Source: CAD feature listing. Evaluate the final solid. Frame: model axes, mm. A direction names the side the tool comes from. Coordinates: 2 decimals unless noted, no trailing zeros. Order: outer loops, then holes, each group sorted by start corner. A loop starts at its lowest first (then second) coordinate and runs counter-clockwise, first axis right, second up.
```python
from build123d import *

# Parameters (mm, degrees)
F0_W      = 72
F0_H      = 24.5
F1_DEPTH  = 18.5
F3_DEPTH  = 11
F3_FACE_R = 14.75
F4_DEPTH  = 19.5
F5_W      = 72
F5_H      = 24.5
F6_DEPTH  = 22.945
F8_DEPTH  = 52.5


with BuildPart() as f1:
    # F0 (on Top) → F1 (new body)
    with BuildSketch(Plane.XY):
        with Locations((36, 12.25)):
            Rectangle(F0_W, F0_H)
    extrude(amount=F1_DEPTH)

    # F2 (on face) → F3 (join)
    with BuildSketch(Plane.YZ.offset(72)):
        with BuildLine():
            ThreePointArc((12.25, 18.5), (22.679825, 22.820175), (27, 33.25))
            ThreePointArc((27, 33.25), (1.820175, 43.679825), (12.25, 18.5))
        make_face()
    extrude(amount=F3_DEPTH)



with BuildPart() as f4:
    # F3_face (on face) → F4 (new body)
    with BuildSketch(Plane(origin=(72, 12.25, 33.25), x_dir=(0, 1, 0), z_dir=(-1, 0, 0))):
        Circle(F3_FACE_R)
    extrude(amount=F4_DEPTH)


with BuildPart() as f1_1:
    add(f1.part)

    add(f4.part)  # F6 merges F4
    # F5 (on face) → F6 (join)
    with BuildSketch(Plane.XY.offset(18.5)):
        with Locations((36, 12.25)):
            Rectangle(F5_W, F5_H)
    extrude(amount=F6_DEPTH)

    # F7 (on face) → F8 (join, through all)
    with BuildSketch(Plane(origin=(0, 0, 0), x_dir=(0, -1, 0), z_dir=(-1, 0, 0))):
        with BuildLine():
            Line((-24.5, 41.445), (0, 41.445))
            ThreePointArc((0, 41.445), (-12.25, 47.995), (-24.5, 41.445))
        make_face()
    extrude(amount=-F8_DEPTH)


solid = f1_1.part
```
1. Draft query along Z for faces 1 (the face through (0, 12, 24)), 2 (the face through (25.882, 12.047, 47.994)), 3 (the face through (35, 12, 0)). Return one class per face: released by +Z, released by -Z, zero draft, split by the parting line, or undercut.
Findings:
face 1: zero draft
face 2: released by +Z
face 3: released by -Z
2. Pin query (flat end, axial travel): P1, Ø6, axis at x = 9.5, y = 10, coming from the +Z side (3 decimals); P2, Ø20.5, axis at x = 53.5, z = 18, coming from the -Y side; P3, Ø10, axis at y = 3.5, z = 12, coming from the +X side. Return the tip coordinate at first contact, or that it passes through.
Findings:
P1: stops at z = 47.995
P2: stops at y = -1.63
P3: stops at x = 72
3. Access query for faces 4 (the face through (35, 24.5, 20)), 5 (the face through (35, 0, 20)), 6 (the face through (83, 12, 33)). Directions: +Z, -Z, +X, -X, +Y, -Y. A direction counts if a zero-diameter tool reaches every point of the face in a straight line with its end or side. Return the directions, or none.
Findings:
face 4: -Z, -X, +Y
face 5: -Z, -X, -Y
face 6: +Z, -Z, +X, +Y, -Y
4. Section query D-D on z = 23. Return loops of the section in (x, y), plus the area to 3 significant figures.
Findings:
outline: (0, 0) - (72, 0) - (72, 1.64) - (83, 1.64) - (83, 22.86) - (72, 22.86) - (72, 24.5) - (0, 24.5) - close
area: 2,000 mm2
5. Section query A-A on z = 14. Return loops of the section in (x, y).
Findings:
outline: (0, 0) - (72, 0) - (72, 24.5) - (0, 24.5) - close
6. Ray query, line 1 (X direction, y = 8.75, z = 3.5); line 2 (Y direction, x = 60, z = 16); line 3 (Z direction, x = 14.5, y = 11.5). Return the intervals inside material, ascending.
Findings:
line 1: x = 0 to 72
line 2: y = 0 to 24.5
line 3: z = 0 to 47.98
7. Section query C-C on x = 6.5. Return loops of the section in (y, z) (3 decimals).
Findings:
outline: (0, 0) - (24.5, 0) - (24.5, 41.445) arc R14.73 ccw to (0, 41.445) - close
